```python
from build123d import *

# Parameters (mm, degrees)
SKETCH1_W           = 320
SKETCH1_H           = 320
SKETCH1_R           = 2.25
SKETCH1_R_2         = 15
SKETCH1_W_2         = 248
SKETCH1_H_2         = 112
BOSS_EXTRUDE1_DEPTH = 3
FILLET1_R           = 10
SKETCH2_R           = 2.25
SKETCH2_R_2         = 15
SKETCH2_W           = 248
SKETCH2_H           = 112
CUT_EXTRUDE1_DEPTH  = 10


with BuildPart() as part:
    # Sketch1 → Boss-Extrude1 (new body)
    with BuildSketch(Plane(origin=(0, 0, 0), x_dir=(1, 0, 0), z_dir=(0, 1, 0))):
        with Locations((45.2, -56.43)):
            Rectangle(SKETCH1_W, SKETCH1_H)
        with Locations((-36.05, -70.43)):
            Circle(SKETCH1_R, mode=Mode.SUBTRACT)
        with Locations((126.45, -70.43)):
            Circle(SKETCH1_R, mode=Mode.SUBTRACT)
        with Locations((128.7, -200.43)):
            Circle(SKETCH1_R, mode=Mode.SUBTRACT)
        with Locations((-33.8, -200.43)):
            Circle(SKETCH1_R, mode=Mode.SUBTRACT)
        with Locations((45.2, -135.43)):
            Circle(SKETCH1_R_2, mode=Mode.SUBTRACT)
        with Locations((45.2, 41.57)):
            Rectangle(SKETCH1_W_2, SKETCH1_H_2, mode=Mode.SUBTRACT)
    extrude(amount=BOSS_EXTRUDE1_DEPTH)

    # Fillet1
    fillet1_edges = [part.edges().sort_by_distance(p)[0] for p in [
        (205.2, 1.5, 216.43),
        (-114.8, 1.5, 216.43),
        (-114.8, 1.5, -103.57),
        (205.2, 1.5, -103.57),
    ]]
    fillet(fillet1_edges, radius=FILLET1_R)

    # Sketch2 → Cut-Extrude1 (cut)
    with BuildSketch(Plane(origin=(0, 3, 0), x_dir=(1, 0, 0), z_dir=(0, 1, 0))):
        with BuildLine():
            Line((-104.8, 99.57), (195.2, 99.57))
            ThreePointArc((195.2, 99.57), (199.442640687, 97.812640687), (201.2, 93.57))
            Line((201.2, 93.57), (201.2, -206.43))
            ThreePointArc((201.2, -206.43), (199.442640687, -210.672640687), (195.2, -212.43))
            Line((195.2, -212.43), (-104.8, -212.43))
            ThreePointArc((-104.8, -212.43), (-109.042640687, -210.672640687), (-110.8, -206.43))
            Line((-110.8, -206.43), (-110.8, 93.57))
            ThreePointArc((-110.8, 93.57), (-109.042640687, 97.812640687), (-104.8, 99.57))
        make_face()
        with Locations((-33.8, -200.43)):
            Circle(SKETCH2_R, mode=Mode.SUBTRACT)
        with Locations((126.45, -70.43)):
            Circle(SKETCH2_R, mode=Mode.SUBTRACT)
        with Locations((-36.05, -70.43)):
            Circle(SKETCH2_R, mode=Mode.SUBTRACT)
        with Locations((128.7, -200.43)):
            Circle(SKETCH2_R, mode=Mode.SUBTRACT)
        with Locations((45.2, -135.43)):
            Circle(SKETCH2_R_2, mode=Mode.SUBTRACT)
        with Locations((45.2, 41.57)):
            Rectangle(SKETCH2_W, SKETCH2_H, mode=Mode.SUBTRACT)
    extrude(amount=-CUT_EXTRUDE1_DEPTH, mode=Mode.SUBTRACT)


solid = part.part
```
Can you work these out from the model? Positions are in its coordinate system, mm. Coordinates: 2 decimals unless noted, no trailing zeros. Write each loop counter-clockwise with the first axis right and the second up, starting at its lowest first coordinate (ties: lowest second). Pieces come first, ordered by that corner, then holes. Notation, with made-up numbers: (-33.5, -17.75) - (-19.5, -17.75) arc R24 cw to (-19.5, 10.25) - close; hole circle Ø7 at (46, 49.25). An arc over 180 degrees is marked (long way). Return JSON: item names as keys, results as strings.
Q1. If we section it at A-A (y = 0.95): Please give me the cut outline in (x, z).
Computed values:
{"outline": "(-114.8, -93.57) arc R10 ccw to (-104.8, -103.57) - (195.2, -103.57) arc R10 ccw to (205.2, -93.57) - (205.2, 206.43) arc R10 ccw to (195.2, 216.43) - (-104.8, 216.43) arc R10 ccw to (-114.8, 206.43) - close; hole (-110.8, -93.57) arc R6 ccw to (-104.8, -99.57) - (195.2, -99.57) arc R6 ccw to (201.2, -93.57) - (201.2, 206.43) arc R6 ccw to (195.2, 212.43) - (-104.8, 212.43) arc R6 ccw to (-110.8, 206.43) - close"}
Q2. If we section it at C-C (x = 141): Please give me the cut outline in (y, z).
Computed values:
{"outline": "(0, -103.57) - (3, -103.57) - (3, -99.57) - (0, -99.57) - close; (0, 212.43) - (3, 212.43) - (3, 216.43) - (0, 216.43) - close"}
Q3. If we section it at B-B (z = 52): Please give me the cut outline in (x, y).
Computed values:
{"outline": "(-114.8, 0) - (-110.8, 0) - (-110.8, 3) - (-114.8, 3) - close; (201.2, 0) - (205.2, 0) - (205.2, 3) - (201.2, 3) - close"}
Q4. Please list where these lines run through material, in increasing order: L1, parallel to X at y = 2.65, z = -8; L2, parallel to Z at x = -88, y = 1.05. Write a range as from..to.
Computed values:
{"L1": "x = -114.8..-110.8, 201.2..205.2", "L2": "z = -103.57..-99.57, 212.43..216.43"}
